Check sheet for the modelled part. Datum: model origin and axes. Units: mm. A direction names the side the tool comes from. Give positions to 0.01 mm unless a question says otherwise; leave off trailing zeros. Loops run counter-clockwise (first coordinate to the right, second up) from the corner with the lowest first, then second, coordinate; pieces in that order, holes last.
Autodesk Fusion 360 part; units mm, degrees
sketch "Sketch1" plane through (0, 0, 0) normal (0, 1, 0) x (1, 0, 0)
  circle A0 centre (0, 0) radius 15
  line L0 (35, 21.25) -> (-35, 21.25)
  line L1 (-35, 21.25) -> (-35, -21.25)
  line L2 (-35, -21.25) -> (35, -21.25)
  line L3 (35, -21.25) -> (35, 21.25)
  line L4 (35, 21.25) -> (-35, -21.25) construction
  line L5 (-35, 21.25) -> (35, -21.25) construction
  line L6 (35, 23.25) -> (-35, 23.25)
  line L7 (-35, 23.25) -> (-35, -23.25)
  line L8 (-35, -23.25) -> (35, -23.25)
  line L9 (35, -23.25) -> (35, 23.25)
  line L10 (35, 23.25) -> (-35, -23.25) construction
  line L11 (-35, 23.25) -> (35, -23.25) construction
  circle A1 centre (0, 0) radius 16
  dimension "d1" = 30
  dimension "d2" = 70
  dimension "d3" = 42.5
  dimension "d4" = 70
  dimension "d5" = 46.5
  dimension "d6" = 32
extrude "Extrude1" add sketch "Sketch1" against normal blind 20 contours A1 makes body 1
extrude "Extrude2" add sketch "Sketch1" against normal blind 2 contours L0 L1 L2 L3 L7 L9 bodies 1
extrude "Extrude3" add sketch "Sketch1" along normal blind 30 separate body contours L0 L6 L7 L9 | L2 L7 L8 L9 makes body 2 at (11.6667, 10, -21.25) makes body 3 at (-11.6667, 10, 23.25)
extrude "Extrude4" add sketch "Sketch1" against normal blind 2 contours L0 L6 L7 L9 | L2 L7 L8 L9 bodies 1 2 3
equation "d4 = d2"
equation "d5 = d3 + 4 mm"
equation "d6 = d1 + 2 mm"
(1) Access from +Z, -Z, +X, -X, +Y, -Y to the whole of each face (thin tool, end or side, straight path). Record for faces 4 (the face through (-3.47, -10.87, 15.62)), 5 (the face through (0, 30, -22)), 6 (the face through (-16, 0, 0)).
(2) Section check A-A on y = 14. Record the boundary of the cut face in (x, z).
(3) Section check D-D on x = 25.5. Record the boundary of the cut face in (y, z).
(4) Material ranges on line 1 (Z direction, x = -0.5, y = 21); line 2 (X direction, y = -10.25, z = 0), recorded low to high.
(5) Section check B-B on x = 0. Record the boundary of the cut face in (y, z).
(6) Gauge pin test, flat ends, axial feed: pin 1 Ø4 at (y, z) = (20.5, -18.5) entering from +X; pin 2 Ø5 at (x, y) = (-14.5, -5) entering from +Z; pin 3 Ø21 at (x, z) = (17, -7.5) entering from +Y. Record the tip position at first contact, or that the pin passes through.
(7) Section check C-C on z = 0. Record the boundary of the cut face in (x, y).
(8) Release check for a two-part mould opening along Z. For faces 1 (the face through (35, -0.3, 1.8)), 2 (the face through (-14.985, -9.86, -0.66)), 3 (the face through (0, 14, -23.25)) record: pulls with the +Z half, pulls with the -Z half, needs draft (parallel to the pull), parting line crosses it, or undercut.
Computed values:
1. face 4: -Y
1. face 5: +Z, -Z, +X, -X, +Y
1. face 6: +X, -X, +Y
2. outline: (-35, -23.25) - (35, -23.25) - (35, -21.25) - (-35, -21.25) - close; (-35, 21.25) - (35, 21.25) - (35, 23.25) - (-35, 23.25) - close
3. outline: (-2, -23.25) - (30, -23.25) - (30, -21.25) - (0, -21.25) - (0, 21.25) - (30, 21.25) - (30, 23.25) - (-2, 23.25) - close
4. line 1: z = -23.25 to -21.25, 21.25 to 23.25
4. line 2: x = -16 to -15, 15 to 16
5. outline: (-20, -16) - (-2, -16) - (-2, -23.25) - (30, -23.25) - (30, -21.25) - (0, -21.25) - (0, -15) - (-20, -15) - close; (-20, 15) - (0, 15) - (0, 21.25) - (30, 21.25) - (30, 23.25) - (-2, 23.25) - (-2, 16) - (-20, 16) - close
6. pin 1: passes through
6. pin 2: stops at z = 10.58
6. pin 3: stops at y = 0
7. outline: (-35, -2) - (-16, -2) - (-16, -20) - (-15, -20) - (-15, 0) - (-35, 0) - close; (15, -20) - (16, -20) - (16, -2) - (35, -2) - (35, 0) - (15, 0) - close
8. face 1: needs draft
8. face 2: undercut
8. face 3: pulls with the -Z half
